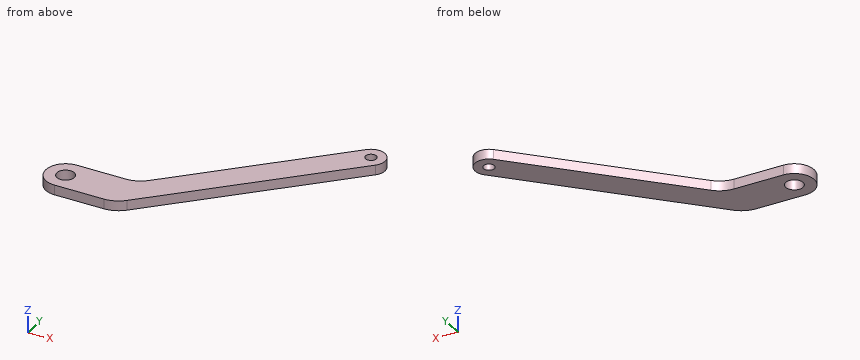
from build123d import *

# Parameters (mm, degrees)
EXTRUDE_1_DEPTH     = 3
SKETCH_9_R          = 2.65
SKETCH_9_R_2        = 1.65
CUT_EXTRUDE_5_DEPTH = 6


with BuildPart() as part:
    # 草图1 → 凸台-拉伸1 (new body)
    with BuildSketch(Plane.XY):
        with BuildLine():
            Line((0.000249999, 5.999750001), (14.999750012, 5.999750001))
            ThreePointArc((14.999750012, 5.999750001), (18.061380786, 6.60878139), (20.656854249, 8.343145751))
            Line((20.656854249, 8.343145751), (63.083261121, 50.769552622))
            ThreePointArc((63.083261121, 50.769552622), (69.093668761, 50.769552622), (69.093668761, 44.759144982))
            Line((69.093668761, 44.759144982), (20.65591759, -3.658290659))
            ThreePointArc((20.65591759, -3.658290659), (18.060942301, -5.391607293), (15.000249999, -6.000249999))
            Line((15.000249999, -6.000249999), (0.000249999, -6.000249999))
            ThreePointArc((0.000249999, -6.000249999), (-5.999750001, -0.000249999), (0.000249999, 5.999750001))
        make_face()
    extrude(amount=EXTRUDE_1_DEPTH)

    # 草图9 → 切除-拉伸5 (cut)
    with BuildSketch(Plane.XY.offset(3)):
        Circle(SKETCH_9_R)
        with Locations((66.088464941, 47.764348802)):
            Circle(SKETCH_9_R_2)
    extrude(amount=-CUT_EXTRUDE_5_DEPTH, mode=Mode.SUBTRACT)


solid = part.part
The model under review builds one solid part; all positions refer to its coordinate system, in mm. Round coordinates to 2 decimals unless told otherwise and drop trailing zeros. Write each loop counter-clockwise with the first axis right and the second up, starting at its lowest first coordinate (ties: lowest second). Pieces come first, ordered by that corner, then holes. Notation, with made-up numbers: (-32, 85.25) -> (-6, 85.25) arc R30 ccw to (-6, 109.25) -> close; hole circle Ø5 at (89.5, 83). An arc over 180 degrees is marked (long way). Answer as a JSON object with one key per item and string values.
1. Clearance check with flat-ended pins moving along their axes: pin 1 (1.5 mm diameter, centred on y = 44, z = 1.5, fed in from -X); pin 2 (1.5 mm diameter, centred on x = 10.5, z = 1, fed in from +Y). State where each tip first meets the part, or that it passes through.
Results found:
{"pin 1": "stops at x = 55.56", "pin 2": "stops at y = 6"}
2. We need section C-C on x = 5.5. State the section outline as (y, z) points, and give its area (3 significant figures).
Results found:
{"outline": "(-6, 0) -> (6, 0) -> (6, 3) -> (-6, 3) -> close", "area": "36.0 mm^2"}
3. We need section A-A on z = 2.15. State the section outline as (x, y) points, and give its area (3 significant figures).
Results found:
{"outline": "(0, -6) -> (15, -6) arc R8 ccw to (20.66, -3.66) -> (69.09, 44.76) arc R4.25 ccw to (63.08, 50.77) -> (20.66, 8.34) arc R8 cw to (15, 6) -> (0, 6) arc R6 ccw to start; hole circle Ø5.3 at (0, 0); hole circle Ø3.3 at (66.09, 47.76)", "area": "848 mm^2"}
4. We need section B-B on y = 0. State the section outline as (x, z) points.
Results found:
{"outline": "(-6, 0) -> (-2.65, 0) -> (-2.65, 3) -> (-6, 3) -> close; (2.65, 0) -> (24.32, 0) -> (24.32, 3) -> (2.65, 3) -> close"}
5. To check wall thickness, follow line 1 along Y through (x, z) = (0, 1.45); line 2 along Y through (x, z) = (9, 0.3); line 3 along X through (y, z) = (1.5, 0.65). State the ranges of each line that lie inside material, in increasing order.
Results found:
{"line 1": "y = -6 to -2.65, 2.65 to 6", "line 2": "y = -6 to 6", "line 3": "x = -5.81 to -2.18, 2.18 to 25.82"}
6. We need section D-D on y = 26.5. State the section outline as (x, z) points, and give its area (3 significant figures).
Results found:
{"outline": "(38.81, 0) -> (50.83, 0) -> (50.83, 3) -> (38.81, 3) -> close", "area": "36.0 mm^2"}
